Build history of the part. All positions in model axes, mm. Give positions to 0.01 mm unless a question says otherwise; leave off trailing zeros. Loops run counter-clockwise (first coordinate to the right, second up) from the corner with the lowest first, then second, coordinate; pieces in that order, holes last. Notation, with made-up numbers: (-6.5, 87.5) -> (18.5, 87.5) arc R21 ccw to (18.5, 118.5) -> close; hole circle Ø9 at (70.25, 45). An arc over 180 degrees is marked (long way). Answer in a Markdown table with one row per item. Add a question column.
from build123d import *

# Parameters (mm, degrees)
SKETCH_1_R               = 4
SKETCH_1_R_2             = 1.6
SKETCH_1_R_3             = 2
SKETCH_1_R_4             = 1.7
F_06_ROTATING_YOKE_DEPTH = 6


with BuildPart() as part:
    # Эскиз1 → 06_Rotating_yoke (new body)
    with BuildSketch(Plane.XY):
        Polygon((-66, -39), (66, -39), (80, -25), (80, 25), (66, 39), (-66, 39), (-80, 25), (-80, -25), align=None)
        Circle(SKETCH_1_R, mode=Mode.SUBTRACT)
        with Locations((-9, 0)):
            Circle(SKETCH_1_R_2, mode=Mode.SUBTRACT)
        with Locations((9, 0)):
            Circle(SKETCH_1_R_2, mode=Mode.SUBTRACT)
        with Locations((0, 9)):
            Circle(SKETCH_1_R_2, mode=Mode.SUBTRACT)
        with Locations((0, -9)):
            Circle(SKETCH_1_R_2, mode=Mode.SUBTRACT)
        with Locations((-68, -25)):
            Circle(SKETCH_1_R_3, mode=Mode.SUBTRACT)
        with Locations((-68, 25)):
            Circle(SKETCH_1_R_3, mode=Mode.SUBTRACT)
        with Locations((68, -25)):
            Circle(SKETCH_1_R_4, mode=Mode.SUBTRACT)
        with Locations((68, 25)):
            Circle(SKETCH_1_R_4, mode=Mode.SUBTRACT)
    extrude(amount=F_06_ROTATING_YOKE_DEPTH)


solid = part.part
(1) Two-plate mould, pull along Y, no slides. Class faces 1 (the cylindrical face through (-10.6, 0.07, 2.96)), 2 (the flat face through (-73, 32, 3)), 3 (the flat face through (-73, -32, 3)): released by +Y, released by -Y, zero draft, split by the parting line, or undercut.
(2) Saw through at C-C, the plane x = -68. List the corners of the cut face in (y, z), then the cut area to 3 significant figures.
(3) Wall check: line 1 along Y through (x, z) = (0, 1.7); line 2 along Y through (x, z) = (68, 4.3); line 3 along Y through (x, z) = (-2.5, 0.35). Give the ranges that are in metal, low to high. Write a range as from..to.
(4) Flat gauge pin, fed straight in: pin 1 Ø2.5 at (x, y) = (68, 25) entering from +Z. Where does the tip first touch, or does it go through?
(5) Saw through at D-D, the plane x = 0. List the corners of the cut face in (y, z), then the cut area to 3 significant figures.
(6) Saw through at B-B, the plane z = 3.35. State how many separate pieces and enclosed holes the cut face has, then the cut area to 3 significant figures.
(7) Saw through at A-A, the plane y = -9. List the corners of the cut face in (x, z).
Worked answers:
| question | item | result |
|---|---|---|
| 1 | face 1 | undercut |
| 1 | face 2 | released by +Y |
| 1 | face 3 | released by -Y |
| 2 | outline | (-37, 0) -> (-27, 0) -> (-27, 6) -> (-37, 6) -> close; (-23, 0) -> (23, 0) -> (23, 6) -> (-23, 6) -> close; (27, 0) -> (37, 0) -> (37, 6) -> (27, 6) -> close |
| 2 | area | 396 mm^2 |
| 3 | line 1 | -39..-10.6, -7.4..-4, 4..7.4, 10.6..39 |
| 3 | line 2 | -37..-26.7, -23.3..23.3, 26.7..37 |
| 3 | line 3 | -39..-3.12, 3.12..39 |
| 4 | pin 1 | through |
| 5 | outline | (-39, 0) -> (-10.6, 0) -> (-10.6, 6) -> (-39, 6) -> close; (-7.4, 0) -> (-4, 0) -> (-4, 6) -> (-7.4, 6) -> close; (4, 0) -> (7.4, 0) -> (7.4, 6) -> (4, 6) -> close; (10.6, 0) -> (39, 0) -> (39, 6) -> (10.6, 6) -> close |
| 5 | area | 382 mm^2 |
| 6 | separate pieces | 1 |
| 6 | enclosed holes | 9 |
| 6 | area | 12,000 mm^2 |
| 7 | outline | (-80, 0) -> (-1.6, 0) -> (-1.6, 6) -> (-80, 6) -> close; (1.6, 0) -> (80, 0) -> (80, 6) -> (1.6, 6) -> close |
